```python
from build123d import *

# Parameters (mm, degrees)
BOSS_EXTRUDE1_DEPTH                  = 76.2
F_12_CLEARANCE_HOLE1_D               = 5.7912
F_12_CLEARANCE_HOLE1_DEPTH           = 68.110147992
F_12_CLEARANCE_HOLE1_TIP             = 1.739852008
F_12_CLEARANCE_HOLE1_ON_FACE_2_D     = 5.7912
F_12_CLEARANCE_HOLE1_ON_FACE_2_DEPTH = 68.110147992
F_12_CLEARANCE_HOLE1_ON_FACE_2_TIP   = 1.739852008


with BuildPart() as part:
    # Sketch1 → Boss-Extrude1 (new body)
    with BuildSketch(Plane.XY):
        with BuildLine():
            Line((0, 0), (38.1, 0))
            ThreePointArc((38.1, 0), (40.34506403, 0.92993597), (41.275, 3.175))
            Line((41.275, 3.175), (41.275, 53.975))
            Line((41.275, 53.975), (38.1, 53.975))
            Line((38.1, 53.975), (38.1, 5.715))
            ThreePointArc((38.1, 5.715), (37.356051224, 3.918948776), (35.56, 3.175))
            Line((35.56, 3.175), (0, 3.175))
            Line((0, 3.175), (0, 0))
        make_face()
    extrude(amount=BOSS_EXTRUDE1_DEPTH)

    # #12 Clearance Hole1
    with Locations(Plane(origin=(41.275, 28.575, 10.16), x_dir=(0, 1, 0), z_dir=(1, 0, 0))):
        with Locations((0, 0), (0, 55.88)):
            Hole(F_12_CLEARANCE_HOLE1_D / 2, depth=F_12_CLEARANCE_HOLE1_DEPTH)
            with Locations((0, 0, -(F_12_CLEARANCE_HOLE1_DEPTH + F_12_CLEARANCE_HOLE1_TIP / 2))):  # 118° drill point
                Cone(0, F_12_CLEARANCE_HOLE1_D / 2, F_12_CLEARANCE_HOLE1_TIP, mode=Mode.SUBTRACT)

    # #12 Clearance Hole1 on face 2
    with Locations(Plane(origin=(17.78, 3.175, 66.04), x_dir=(0, 0, 1), z_dir=(0, 1, 0))):
        with Locations((0, 0), (-55.88, 0)):
            Hole(F_12_CLEARANCE_HOLE1_ON_FACE_2_D / 2, depth=F_12_CLEARANCE_HOLE1_ON_FACE_2_DEPTH)
            with Locations((0, 0, -(F_12_CLEARANCE_HOLE1_ON_FACE_2_DEPTH + F_12_CLEARANCE_HOLE1_ON_FACE_2_TIP / 2))):  # 118° drill point
                Cone(0, F_12_CLEARANCE_HOLE1_ON_FACE_2_D / 2, F_12_CLEARANCE_HOLE1_ON_FACE_2_TIP, mode=Mode.SUBTRACT)


solid = part.part
```
Geometry check sheet. Reference: the model listing, model coordinates, mm. A direction names the side the tool comes from. Give positions to 0.01 mm unless a question says otherwise; leave off trailing zeros. Order: outer loops, then holes, each group sorted by start corner. A loop starts at its lowest first (then second) coordinate and runs counter-clockwise, first axis right, second up. Notation, with made-up numbers: (4, -25) -> (10, -25) arc R25 ccw to (10, 4) -> close; hole circle Ø1 at (56.25, 60.25). An arc over 180 degrees is marked (long way). Write each question's results on one line, items separated by ' | '. Start each with the question number.
(1) Scan lines: line 1 (Z direction, x = 17, y = 1); line 2 (X direction, y = 20.5, z = 28) (3 decimals); line 3 (Y direction, x = 35, z = 7) (3 decimals). Record each from-to range of solid material in increasing order.
(2) Sectioned sample at D-D (y = 8). Enter the section's corners in (x, z) (3 decimals), plus the area to 3 significant figures.
(3) Sectioned sample at C-C (z = 42). Enter the section's corners in (x, y) (3 decimals).
(4) Access from +Z, -Z, +X, -X, +Y, -Y to the whole of each face (thin tool, end or side, straight path). Record for faces 4 (the face through (38.1, 30, 38)), 5 (the face through (39.67, 28.95, 68.91)).
(5) Sectioned sample at A-A (z = 66.04). Enter the section's corners in (x, y) (3 decimals), plus the area to 3 significant figures.
(6) Gauge pin test, flat ends, axial feed: P1, Ø6.5, axis at y = 28.575, z = 66.04, coming from the -X side; P2, Ø5, axis at x = 17.78, z = 10.16, coming from the +Y side; P3, Ø5, axis at x = 21, z = 23, coming from the +Y side (3 decimals). Record the tip position at first contact, or that the pin passes through.
(7) Sectioned sample at B-B (x = 17.78). Enter the section's corners in (y, z) (3 decimals).
(8) Mould release check, pull along Z, two halves, no side actions. Record for faces 1 (the face through (14.953, 1.565, 10.788)), 2 (the face through (39, 15, 0)), 3 (the face through (19, 0, 38)): pulls with the +Z half, pulls with the -Z half, needs draft (parallel to the pull), parting line crosses it, or undercut.
Answer below:
1) line 1: 0 to 7.37, 12.95 to 63.25, 68.83 to 76.2 | line 2: 38.1 to 41.275 | line 3: 0 to 3.175
2) outline: (38.1, 0) -> (41.275, 0) -> (41.275, 76.2) -> (38.1, 76.2) -> close | area: 242 mm2
3) outline: (0, 0) -> (38.1, 0) arc R3.175 ccw to (41.275, 3.175) -> (41.275, 53.975) -> (38.1, 53.975) -> (38.1, 5.715) arc R2.54 cw to (35.56, 3.175) -> (0, 3.175) -> close
4) face 4: +Z, -Z, -X, +Y | face 5: +X, -X
5) outline: (0, 0) -> (14.884, 0) -> (14.884, 3.175) -> (0, 3.175) -> close; (20.676, 0) -> (38.1, 0) arc R3.175 ccw to (41.275, 3.175) -> (41.275, 25.679) -> (38.1, 25.679) -> (38.1, 5.715) arc R2.54 cw to (35.56, 3.175) -> (20.676, 3.175) -> close; (38.1, 31.471) -> (41.275, 31.471) -> (41.275, 53.975) -> (38.1, 53.975) -> close | area: 255 mm2
6) P1: x = 38.1 | P2: through | P3: y = 3.175
7) outline: (0, 0) -> (3.175, 0) -> (3.175, 7.264) -> (0, 7.264) -> close; (0, 13.056) -> (3.175, 13.056) -> (3.175, 63.144) -> (0, 63.144) -> close; (0, 68.936) -> (3.175, 68.936) -> (3.175, 76.2) -> (0, 76.2) -> close
8) face 1: undercut | face 2: pulls with the -Z half | face 3: needs draft
